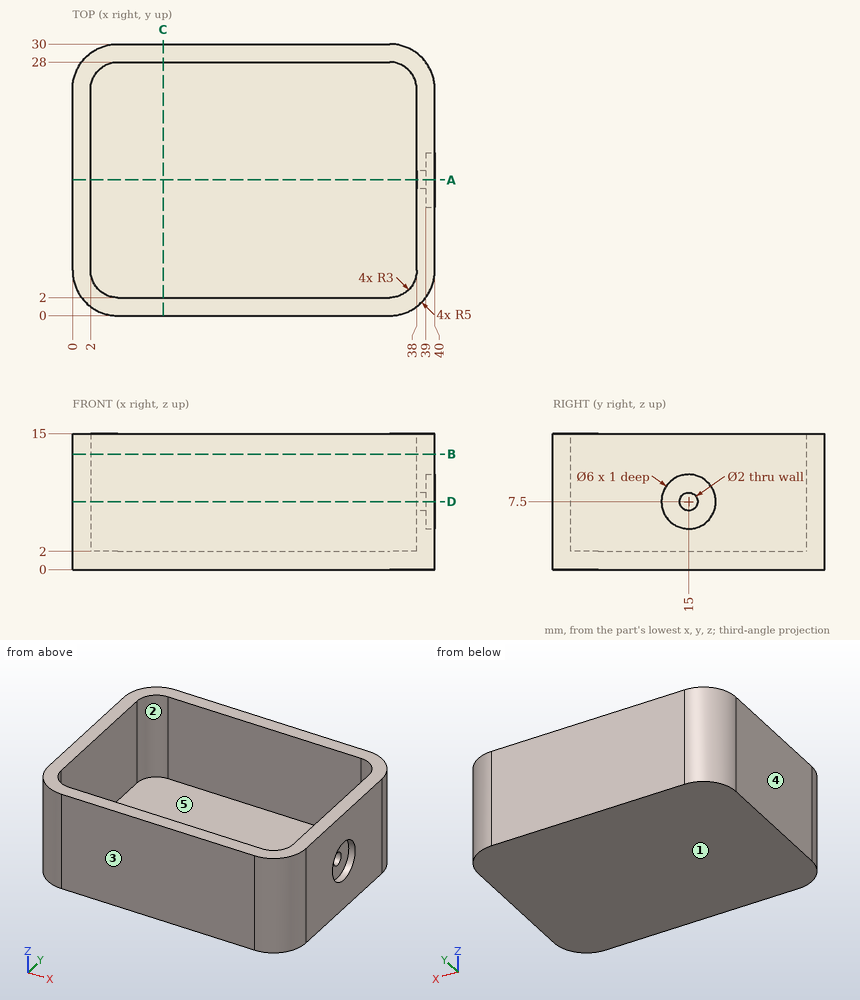
Can you work these out from the drawing? Everything is in mm from the part's minimum corner. A direction names the side the tool comes from. Give positions to 0.01 mm unless a question says otherwise; leave off trailing zeros. Loops run counter-clockwise (first coordinate to the right, second up) from the corner with the lowest first, then second, coordinate; pieces in that order, holes last. Notation, with made-up numbers: (56, -6.5) -> (98, -6.5) arc R34 cw to (98, 23.5) -> close; hole circle Ø1 at (45, 7.5). An arc over 180 degrees is marked (long way). Write item = value, one per line.
1) Suppose I cut it at A-A on y = 15. Write out the boundary of the cut face in (x, z), then the cut area to 3 significant figures.
Check result:
outline = (0, 0) -> (40, 0) -> (40, 4.5) -> (39, 4.5) -> (39, 6.5) -> (38, 6.5) -> (38, 2) -> (2, 2) -> (2, 15) -> (0, 15) -> close; (38, 8.5) -> (39, 8.5) -> (39, 10.5) -> (40, 10.5) -> (40, 15) -> (38, 15) -> close
area = 124 mm2
2) I need wall thicknesses on L1, parallel to Y at x = 17.5, z = 10.75; L2, parallel to X at y = 24.5, z = 3.5; L3, parallel to Z at x = 38.8, y = 15. Which ranges of each line are inside material? Lowest first, please. Write a range as from..to.
Check result:
L1 = 0..2, 28..30
L2 = 0..2, 38..40
L3 = 0..6.5, 8.5..15
3) Suppose I cut it at D-D on z = 7.5. Write out the boundary of the cut face in (x, y).
Check result:
outline = (0, 5) arc R5 ccw to (5, 0) -> (35, 0) arc R5 ccw to (40, 5) -> (40, 12) -> (39, 12) -> (39, 14) -> (38, 14) -> (38, 5) arc R3 cw to (35, 2) -> (5, 2) arc R3 cw to (2, 5) -> (2, 25) arc R3 cw to (5, 28) -> (35, 28) arc R3 cw to (38, 25) -> (38, 16) -> (39, 16) -> (39, 18) -> (40, 18) -> (40, 25) arc R5 ccw to (35, 30) -> (5, 30) arc R5 ccw to (0, 25) -> close
4) Suppose I cut it at B-B on z = 12.75. Write out the boundary of the cut face in (x, y), then the cut area to 3 significant figures.
Check result:
outline = (0, 5) arc R5 ccw to (5, 0) -> (35, 0) arc R5 ccw to (40, 5) -> (40, 25) arc R5 ccw to (35, 30) -> (5, 30) arc R5 ccw to (0, 25) -> close; hole (2, 5) arc R3 ccw to (5, 2) -> (35, 2) arc R3 ccw to (38, 5) -> (38, 25) arc R3 ccw to (35, 28) -> (5, 28) arc R3 ccw to (2, 25) -> close
area = 250 mm2
5) Will these pins go through, and if not, where does the flat tip stop? pin 1 (13 mm diameter, centred on x = 26, y = 10.5, fed in from +Z); pin 2 (6.5 mm diameter, centred on y = 15.5, z = 6.5, fed in from +X); pin 3 (1.8 mm diameter, centred on y = 15, z = 7.5, fed in from +X).
Check result:
pin_1 = 2
pin_2 = 40
pin_3 = 2
6) Thinking about a two-plate mould opening in X: for the marked faces 3, 4 and 5, which applies, released by +X, released by -X, zero draft, split by the parting line, or undercut?
Check result:
face_3 = zero draft
face_4 = released by -X
face_5 = undercut
7) For the marked faces 1 and 2, which set-ups out of +Z, -Z, +X, -X, +Y, -Y let a thin tool reach every point of the face, with its end or its side?
Check result:
face_1 = -Z, +X, -X, +Y, -Y
face_2 = +Z
8) Suppose I cut it at C-C on x = 10. Write out the boundary of the cut face in (y, z), then the cut area to 3 significant figures.
Check result:
outline = (0, 0) -> (30, 0) -> (30, 15) -> (28, 15) -> (28, 2) -> (2, 2) -> (2, 15) -> (0, 15) -> close
area = 112 mm2
